from build123d import *

# Parameters (mm, degrees)
SKETCH3_R          = 3
CUT_EXTRUDE1_DEPTH = 90.582364336


with BuildPart() as part:
    # Sketch1 → Revolve1 (revolve)
    with BuildSketch(Plane.XY, mode=Mode.PRIVATE) as revolve1_sk:
        Polygon((20, 50), (27.5, 50), (27.5, 6), (-27.5, 6), (-27.5, 50), (-20, 50), (-20, 44), (20, 44), align=None)
    revolve(revolve1_sk.sketch.rotate(Axis((-137.236084453, 0, 0), (1, 0, 0)), 90), axis=Axis((-137.236084453, 0, 0), (1, 0, 0)))

    # Sketch3 → Cut-Extrude1 (cut, through all)
    with BuildSketch(Plane(origin=(27.5, 0, 0), x_dir=(0, 0, -1), z_dir=(1, 0, 0))):
        with Locations((0, 25)):
            Circle(SKETCH3_R)
        with Locations((0, -25)):
            Circle(SKETCH3_R)
    extrude(amount=-CUT_EXTRUDE1_DEPTH, mode=Mode.SUBTRACT)


solid = part.part
Model file for the job. Use its own axes, mm. A direction names the side the tool comes from. Give positions to 0.01 mm unless a question says otherwise; leave off trailing zeros. Order: outer loops, then holes, each group sorted by start corner. A loop starts at its lowest first (then second) coordinate and runs counter-clockwise, first axis right, second up. Notation, with made-up numbers: (32, 20) - (57, 20) arc R37 ccw to (57, 57) - close; hole circle Ø7 at (24.5, 87). An arc over 180 degrees is marked (long way). Return JSON: item names as keys, results as strings.
1) Cut at C-C, the plane x = 23. Give the cut face in (y, z), plus the area to 3 significant figures.
Geometry says:
{"outline": "circle Ø100 at (0, 0); hole circle Ø6 at (-25, 0); hole circle Ø12 at (0, 0); hole circle Ø6 at (25, 0)", "area": "7,680 mm²"}
2) Cut at A-A, the plane z = 0. Give the cut face in (x, y), plus the area to 3 significant figures.
Geometry says:
{"outline": "(-27.5, -50) - (-20, -50) - (-20, -44) - (20, -44) - (20, -50) - (27.5, -50) - (27.5, -28) - (-27.5, -28) - close; (-27.5, -22) - (27.5, -22) - (27.5, -6) - (-27.5, -6) - close; (-27.5, 6) - (27.5, 6) - (27.5, 22) - (-27.5, 22) - close; (-27.5, 28) - (27.5, 28) - (27.5, 50) - (20, 50) - (20, 44) - (-20, 44) - (-20, 50) - (-27.5, 50) - close", "area": "3,700 mm²"}
3) Pull direction Z, two halves, no side cores. Call faces 3 (the cylindrical face through (0.39, -27.93, 0.65)), 4 (the flat face through (27.5, 10, -1)), 5 (the cylindrical face through (0.28, 42.954, -9.538)), 6 (the cylindrical face through (0.39, 22.07, 0.65)): pulls with the +Z half, pulls with the -Z half, needs draft (parallel to the pull), parting line crosses it, or undercut.
Geometry says:
{"face 3": "undercut", "face 4": "needs draft", "face 5": "parting line crosses it", "face 6": "undercut"}
4) Flat gauge pins, fed straight in: P1, Ø4, axis at x = -6, y = 40, coming from the -Z side; P2, Ø2, axis at x = 12, y = -31.5, coming from the +Z side; P3, Ø5.5, axis at y = 25, z = 0, coming from the -X side; P4, Ø3, axis at x = -0.5, y = 29, coming from the -Z side. Where does each tip first touch, or does it go through?
Geometry says:
{"P1": "z = -22.18", "P2": "z = 31.71", "P3": "through", "P4": "z = -34.35"}
5) Probe line 1 (Y direction, x = -6, z = 0); line 2 (Z direction, x = -1.5, y = -0.5); line 3 (X direction, y = -41.5, z = 19). List the from-to ranges inside material, lowest first. Write a range as from..to.
Geometry says:
{"line 1": "-44..-28, -22..-6, 6..22, 28..44", "line 2": "-44..-5.98, 5.98..44", "line 3": "-27.5..-20, 20..27.5"}
6) 3-axis set-ups, long thin cutter, end or side, ignore diameter. For faces 1 (the flat face through (-20, 44.2, -0.2)), 2 (the cylindrical face through (-23.7, -15.02, 47.69)): which of +Z, -Z, +X, -X, +Y, -Y reach the whole face in a straight line?
Geometry says:
{"face 1": "none", "face 2": "+X, -X"}
7) Cut at D-D, the plane y = -25. Give the cut face in (x, z).
Geometry says:
{"outline": "(-27.5, -43.3) - (-20, -43.3) - (-20, -36.21) - (20, -36.21) - (20, -43.3) - (27.5, -43.3) - (27.5, -3) - (-27.5, -3) - close; (-27.5, 3) - (27.5, 3) - (27.5, 43.3) - (20, 43.3) - (20, 36.21) - (-20, 36.21) - (-20, 43.3) - (-27.5, 43.3) - close"}
8) Cut at B-B, the plane y = 0. Give the cut face in (x, z), plus the area to 3 significant figures.
Geometry says:
{"outline": "(-27.5, -50) - (-20, -50) - (-20, -44) - (20, -44) - (20, -50) - (27.5, -50) - (27.5, -6) - (-27.5, -6) - close; (-27.5, 6) - (27.5, 6) - (27.5, 50) - (20, 50) - (20, 44) - (-20, 44) - (-20, 50) - (-27.5, 50) - close", "area": "4,360 mm²"}
